Part model, mm, in its own coordinate system. Round coordinates to 2 decimals unless told otherwise and drop trailing zeros. Loops run counter-clockwise (first coordinate to the right, second up) from the corner with the lowest first, then second, coordinate; pieces in that order, holes last. Notation, with made-up numbers: (-28, 11.5) -> (20, 11.5) arc R18 ccw to (20, 45.5) -> close; hole circle Ø6 at (27, 53). An arc over 180 degrees is marked (long way). Answer as CSV lines item,"result".
from build123d import *

# Parameters (mm, degrees)
SKETCH1_R           = 3.8
SKETCH1_R_2         = 3.3
BOSS_EXTRUDE2_DEPTH = 76
SKETCH2_W           = 1
SKETCH2_H           = 5
CUT_EXTRUDE4_DEPTH  = 8
CIRPATTERN1_COUNT   = 3
SCALE2_SCALE        = 10


with BuildPart() as part:
    # Sketch1 → Boss-Extrude2 (new body)
    with BuildSketch(Plane(origin=(0, 0, 0), x_dir=(1, 0, 0), z_dir=(0, 1, 0))):
        with Locations(Location((0, 0, 0), (0, 0, 270))):
            Circle(SKETCH1_R)
        with Locations(Location((0, 0, 0), (0, 0, 270))):
            Circle(SKETCH1_R_2, mode=Mode.SUBTRACT)
    extrude(amount=BOSS_EXTRUDE2_DEPTH)

    # Sketch2 → Cut-Extrude4 (cut)
    with BuildSketch(Plane.XY):
        with Locations((0, 6.5)):
            Rectangle(SKETCH2_W, SKETCH2_H)
    cut_extrude4 = extrude(amount=CUT_EXTRUDE4_DEPTH, mode=Mode.SUBTRACT)

    # CirPattern1: Cut-Extrude4 ×3 about axis
    cirpattern1_axis = Axis((0, 0, 0), (0, 1, 0))
    for i in range(1, CIRPATTERN1_COUNT):
        add(cut_extrude4.rotate(cirpattern1_axis, i * 360 / CIRPATTERN1_COUNT), mode=Mode.SUBTRACT)


with BuildPart() as part_1:
    # Scale2: scaled about (0, 0, 0)
    add(part.part.scale(SCALE2_SCALE))


solid = part_1.part
Q1. Two-plate mould, pull along X, no slides. Class faces 1 (the face through (-23.122, 374.68, -30.156)), 2 (the face through (-32.215, 374.68, -7.154)), 3 (the face through (31.14, 0, -11.44)): pulls with the +X half, pulls with the -X half, needs draft (parallel to the pull), parting line crosses it, or undercut.
Geometry results:
face 1,"parting line crosses it"
face 2,"undercut"
face 3,"needs draft"
Q2. Saw through at C-C, the plane x = -18.5. Write the cut outline in (y, z).
Geometry results:
outline,"(0, -33.19) -> (760, -33.19) -> (760, -27.33) -> (0, -27.33) -> close; (0, 27.33) -> (760, 27.33) -> (760, 33.19) -> (0, 33.19) -> close"
Q3. Saw through at A-A, the plane z = 0. Write the cut outline in (x, y), then the cut area to 3 significant figures.
Geometry results:
outline,"(-38, 0) -> (-33, 0) -> (-33, 760) -> (-38, 760) -> close; (33, 0) -> (38, 0) -> (38, 760) -> (33, 760) -> close"
area,"7,600 mm2"
Q4. Drill centre lines: line 1 along X through (y, z) = (583, 0); line 2 along X through (y, z) = (373, 2); line 3 along Z through (x, y) = (16, 204). Where is each one in solid material? Low to high.
Geometry results:
line 1,"-38 to -33, 33 to 38"
line 2,"-37.95 to -32.94, 32.94 to 37.95"
line 3,"-34.47 to -28.86, 28.86 to 34.47"
Q5. Saw through at B-B, the plane y = 48.5. Write the cut outline in (x, z), then the cut area to 3 significant figures.
Geometry results:
outline,"(-35.12, -14.5) -> (-30.75, -11.98) arc R33 cw to (-5, 32.62) -> (-5, 37.67) arc R38 ccw to start; (-30.12, -23.16) arc R38 ccw to (30.12, -23.16) -> (25.75, -20.64) arc R33 cw to (-25.75, -20.64) -> close; (5, 32.62) arc R33 cw to (30.75, -11.98) -> (35.12, -14.5) arc R38 ccw to (5, 37.67) -> close"
area,"965 mm2"
Q6. Saw through at D-D, the plane y = 231. Write the cut outline in (x, z).
Geometry results:
outline,"circle Ø76 at (0, 0); hole circle Ø66 at (0, 0)"
Q7. Drop flat-ended pins along their axis: P1, Ø12, axis at y = 631.5, z = 20, coming from the -X side; P2, Ø2.5, axis at y = 73, z = 36, coming from the -X side; P3, Ø4, axis at x = -19.5, y = 482.5, coming from the +Z side. Give the stop position or say it passes through.
Geometry results:
P1,"x = -35.33"
P2,"x = -15.38"
P3,"z = 33.73"
